Geometry check sheet. Reference: drawing and pictorial views, mm from the part's lowest x, y, z. A direction names the side the tool comes from. Give positions to 0.01 mm unless a question says otherwise; leave off trailing zeros. Order: outer loops, then holes, each group sorted by start corner. A loop starts at its lowest first (then second) coordinate and runs counter-clockwise, first axis right, second up.
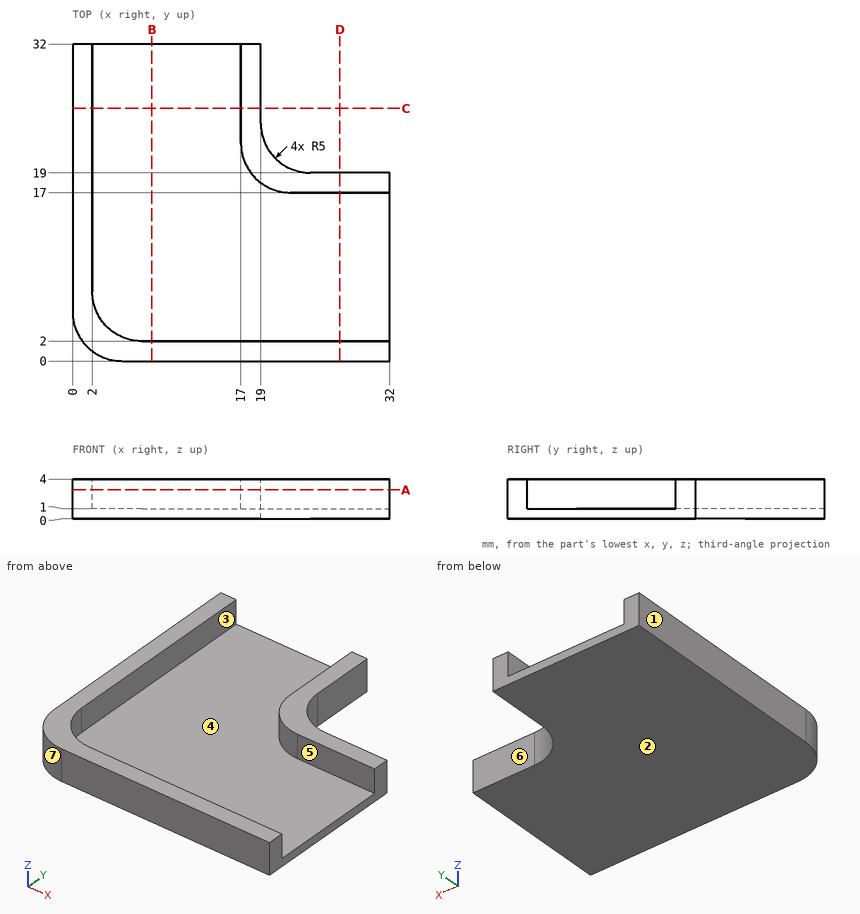
(1) Set-up check for the marked faces 4, 5, 6 and 7: record each of +Z, -Z, +X, -X, +Y, -Y from which the full face is reachable in a straight line by a thin tool's end or side.
Response values:
face 4: +Z
face 5: +Z, +X
face 6: +Z, -Z, +X, +Y
face 7: +Z, -Z, -X, -Y
(2) Release check for a two-part mould opening along X. For the marked faces 1, 2 and 3 record: released by +X, released by -X, zero draft, split by the parting line, or undercut.
Response values:
face 1: released by -X
face 2: zero draft
face 3: undercut
(3) Cross-section at C-C on y = 25.5. Enter the section's corners in (x, z), then the cut area to 3 significant figures.
Response values:
outline: (0, 0) - (19, 0) - (19, 4) - (17, 4) - (17, 1) - (2, 1) - (2, 4) - (0, 4) - close
area: 31.0 mm2
(4) Material ranges on L1, parallel to Y at x = 25.5, z = 2; L2, parallel to Z at x = 10, y = 26; L3, parallel to Y at x = 11, z = 3, recorded low to high.
Response values:
L1: y = 0 to 2, 17 to 19
L2: z = 0 to 1
L3: y = 0 to 2
(5) Gauge pin test, flat ends, axial feed: pin 1 Ø1.5 at (x, y) = (7, 16.5) entering from +Z; pin 2 Ø1.5 at (x, z) = (24.5, 3) entering from +Y; pin 3 Ø1.5 at (x, z) = (16, 2.5) entering from +Y. Record the tip position at first contact, or that the pin passes through.
Response values:
pin 1: stops at z = 1
pin 2: stops at y = 19.01
pin 3: stops at y = 2
(6) Cross-section at B-B on x = 8. Enter the section's corners in (y, z), then the cut area to 3 significant figures.
Response values:
outline: (0, 0) - (32, 0) - (32, 1) - (2, 1) - (2, 4) - (0, 4) - close
area: 38.0 mm2
(7) Cross-section at A-A on z = 2.9. Enter the section's corners in (x, y).
Response values:
outline: (0, 5) arc R5 ccw to (5, 0) - (32, 0) - (32, 2) - (7, 2) arc R5 cw to (2, 7) - (2, 32) - (0, 32) - close; (17, 22) arc R5 ccw to (22, 17) - (32, 17) - (32, 19) - (24, 19) arc R5 cw to (19, 24) - (19, 32) - (17, 32) - close
